Geometry: final body of the model. Coordinates: model frame, mm. Face numbers are marked on the shaded views. A direction names the side the tool comes from. Give positions to 0.01 mm unless a question says otherwise; leave off trailing zeros. Order: outer loops, then holes, each group sorted by start corner. A loop starts at its lowest first (then second) coordinate and runs counter-clockwise, first axis right, second up. Notation, with made-up numbers: (1.25, 39.5) - (36.25, 39.5) arc R24 cw to (36.25, 77.5) - close; hole circle Ø8 at (14, 47.25). An arc over 180 degrees is marked (long way). Put each result on its own line as item: value. Start each with the question number.
1. Section A-A on y = -39. Return the cut outline in (x, z).
2. First-contact query: P1, Ø10, axis at x = -11, z = -12, coming from the -Y side; P2, Ø14.5, axis at y = 7.5, z = -15, coming from the +X side; P3, Ø3, axis at x = -12, y = -2.5, coming from the -Z side. Flat tips, straight axial feed; report the tip coordinate or a pass-through.
3. Mould query, pull axis X, two halves, no side actions, for the marked faces 5, 6 and 7. Classes: pulls with the +X half, pulls with the -X half, needs draft (parallel to the pull), parting line crosses it, or undercut.
4. Ray query, line 1 along X through (y, z) = (-39, -12.5); line 2 along Z through (x, y) = (4.5, -36); line 3 along X through (y, z) = (-2, -11). Return the intervals inside material, ascending. Write a range as from..to.
5. Section D-D on y = 0. Return the cut outline in (x, z), plus the area to 3 significant figures.
6. Section B-B on x = 11.5. Return the cut outline in (y, z).
7. Section C-C on z = 9. Return the cut outline in (x, y), plus the area to 3 significant figures.
8. Set-up query: the marked faces 1, 2, 3 and 4. Return all of +Z, -Z, +X, -X, +Y, -Y with unobstructed straight access to the full face (end or side cutting, diameter ignored); none if empty.
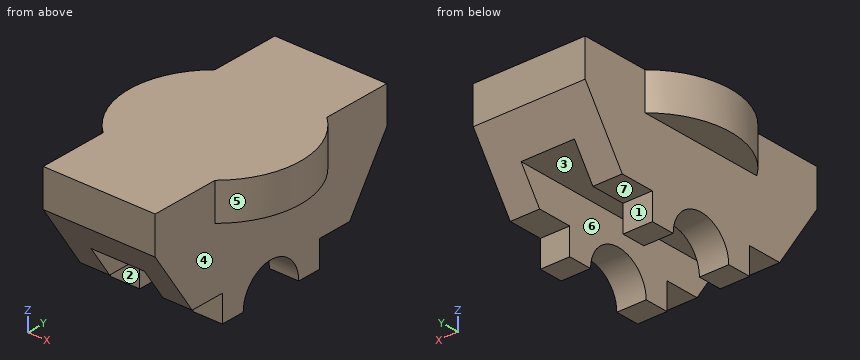
from build123d import *

# Parameters (mm, degrees)
SKETCH1_W           = 42
SKETCH1_H           = 100
BOSS_EXTRUDE2_DEPTH = 14
BOSS_EXTRUDE3_DEPTH = 14
BOSS_EXTRUDE4_DEPTH = 11
SKETCH11_W          = 20
SKETCH11_H          = 12
BOSS_EXTRUDE5_DEPTH = 100
CUT_EXTRUDE1_DEPTH  = 74.620649277


with BuildPart() as part:
    # Sketch1 → Boss-Extrude2 (new body)
    with BuildSketch(Plane.XY):
        Rectangle(SKETCH1_W, SKETCH1_H)
    extrude(amount=BOSS_EXTRUDE2_DEPTH)

    # Sketch3 → Boss-Extrude3 (add)
    with BuildSketch(Plane.XY.offset(14)):
        with BuildLine():
            Line((-21, 24.145392935), (-21, -24.145392935))
            ThreePointArc((-21, -24.145392935), (-32, 0), (-21, 24.145392935))
        make_face()
        with BuildLine():
            Line((21, 24.145392935), (21, -24.145392935))
            ThreePointArc((21, -24.145392935), (32, 0), (21, 24.145392935))
        make_face()
    extrude(amount=-BOSS_EXTRUDE3_DEPTH)

    # Sketch4 → Boss-Extrude4 (add)
    with BuildSketch(Plane(origin=(21, 0, 0), x_dir=(0, 0, -1), z_dir=(1, 0, 0))):
        with BuildLine():
            Line((34, 12), (34, 21))
            Line((34, 21), (24, 21))
            Line((24, 21), (24, 34))
            Line((24, 34), (0, 50))
            Line((0, 50), (0, -50))
            Line((0, -50), (24, -34))
            Line((24, -34), (24, -21))
            Line((24, -21), (34, -21))
            Line((34, -21), (34, -12))
            ThreePointArc((34, -12), (22, 0), (34, 12))
        make_face()
    boss_extrude4 = extrude(amount=-BOSS_EXTRUDE4_DEPTH)

    # Mirror1: Boss-Extrude4 across plane
    add(boss_extrude4.mirror(Plane(origin=(0, 0, 0), x_dir=(0, 0, 1), z_dir=(1, 0, 0))))

    # Sketch11 → Boss-Extrude5 (add, through all)
    with BuildSketch(Plane(origin=(0, 50, 0), x_dir=(1, 0, 0), z_dir=(0, 1, 0))):
        with Locations((0, 6)):
            Rectangle(SKETCH11_W, SKETCH11_H)
    extrude(amount=-BOSS_EXTRUDE5_DEPTH)

    # Sketch12 → Cut-Extrude1 (cut, through all)
    with BuildSketch(Plane(origin=(10, 0, 0), x_dir=(0, 0, -1), z_dir=(1, 0, 0))):
        Polygon((0, 50), (12, 42), (12, 50), align=None)
    cut_extrude1 = extrude(amount=-CUT_EXTRUDE1_DEPTH, mode=Mode.SUBTRACT)

    # Mirror2: Cut-Extrude1 across plane
    add(cut_extrude1.mirror(Plane.ZX), mode=Mode.SUBTRACT)


solid = part.part
Resolved:
1. outline: (-21, -16.5) - (-10, -16.5) - (-10, -12) - (10, -12) - (10, -16.5) - (21, -16.5) - (21, 14) - (-21, 14) - close
2. P1: y = -45.33
2. P2: x = 21
2. P3: z = -22.69
3. face 5: pulls with the +X half
3. face 6: undercut
3. face 7: needs draft
4. line 1: -21..-10, 10..21
4. line 2: -12..14
4. line 3: -21..21
5. outline: (-32, 0) - (-21, 0) - (-21, -22) - (-10, -22) - (-10, -12) - (10, -12) - (10, -22) - (21, -22) - (21, 0) - (32, 0) - (32, 14) - (-32, 14) - close
5. area: 1,620 mm^2
6. outline: (-50, 0) - (-34, -24) - (-21, -24) - (-21, -34) - (-12, -34) arc R12 cw to (12, -34) - (21, -34) - (21, -24) - (34, -24) - (50, 0) - (50, 14) - (-50, 14) - close
7. outline: (-21, -50) - (21, -50) - (21, -24.15) arc R32 ccw to (21, 24.15) - (21, 50) - (-21, 50) - (-21, 24.15) arc R32 ccw to (-21, -24.15) - close
7. area: 4,940 mm^2
8. face 1: -Z, +X, -X, +Y
8. face 2: -Z, +X, -X, -Y
8. face 3: -Z, +Y, -Y
8. face 4: -Z, +X
